from build123d import *

# Parameters (mm, degrees)
F0_W     = 209.55
F0_H     = 88.9
F1_DEPTH = 3.175
F2_W     = 44.45
F2_H     = 3.175
F3_DEPTH = 25.4
F4_W     = 6.35
F4_H     = 4.7625
F5_DEPTH = 3.175


# Not quite as in the source:
# - a length typed as a fraction of an inch, garbled in the dataset ("3 / 203.2 mm" for 3/8 in), is restored


with BuildPart() as f1:
    # F0 (on Top) → F1 (new body)
    with BuildSketch(Plane.XY):
        Rectangle(F0_W, F0_H)
    extrude(amount=F1_DEPTH)

    # F2 (on face) → F3 (cut)
    with BuildSketch(Plane.XY.offset(3.175)):
        with Locations((-82.55, -30.1625)):
            Rectangle(F2_W, F2_H)
        with Locations((82.55, -30.1625)):
            Rectangle(F2_W, F2_H)
        with Locations((0, -30.1625)):
            Rectangle(F2_W, F2_H)
    extrude(amount=-F3_DEPTH, mode=Mode.SUBTRACT)

    # F4 (on face) → F5 (join)
    with BuildSketch(Plane.XY.offset(3.175)):
        with Locations((-88.9, 46.83125)):
            Rectangle(F4_W, F4_H)
        with Locations((88.9, 46.83125)):
            Rectangle(F4_W, F4_H)
    extrude(amount=-F5_DEPTH)


solid = f1.part
Source: CAD feature listing. Evaluate the final solid. Frame: model axes, mm. Coordinates: 2 decimals unless noted, no trailing zeros. Write each loop counter-clockwise with the first axis right and the second up, starting at its lowest first coordinate (ties: lowest second). Pieces come first, ordered by that corner, then holes. Notation, with made-up numbers: M 23,70.25 L 43,70.25 A22 ccw 43,90.25 Z; hole C 30,-19.5 d5. An arc over 180 degrees is marked long. Use a Markdown table: item, result.
1) Section A-A, the plane x = 11. Output: boundary loops of the cut face in (y, z) (3 decimals).
Conclusion:
| item | result |
|---|---|
| outline | M -44.45,0 L -31.75,0 L -31.75,3.175 L -44.45,3.175 Z; M -28.575,0 L 44.45,0 L 44.45,3.175 L -28.575,3.175 Z |
2) Section C-C, the plane x = 47.5. Output: boundary loops of the cut face in (y, z) (3 decimals), then the cut area to 3 significant figures.
Conclusion:
| item | result |
|---|---|
| outline | M -44.45,0 L 44.45,0 L 44.45,3.175 L -44.45,3.175 Z |
| area | 282 mm^2 |
3) First-contact query: pin 1 Ø1.6 at (y, z) = (46.5, 1.5) entering from +X (3 decimals); pin 2 Ø3 at (x, y) = (-79.5, 21) entering from -Z; pin 3 Ø1.6 at (x, z) = (1, 2) entering from +Y; pin 4 Ø1.6 at (y, z) = (-30.5, 2) entering from -X (3 decimals). Flat tips, straight axial feed; report the tip coordinate or a pass-through.
Conclusion:
| item | result |
|---|---|
| pin 1 | stops at x = 92.075 |
| pin 2 | stops at z = 0 |
| pin 3 | stops at y = 44.45 |
| pin 4 | stops at x = -60.325 |
4) Ray query, L1, parallel to Y at x = -13.5, z = 1.2 (3 decimals); L2, parallel to Y at x = -30.5, z = 1.4. Return the intervals inside material, ascending.
Conclusion:
| item | result |
|---|---|
| L1 | y = -44.45 to -31.75, -28.575 to 44.45 |
| L2 | y = -44.45 to 44.45 |
